from build123d import *

# Parameters (mm, degrees)
SKETCH1_R           = 2.5
BOSS_EXTRUDE1_DEPTH = 25
SKETCH2_W           = 2
SKETCH2_H           = 3
SKETCH2_W_2         = 1
SKETCH2_H_2         = 2
BOSS_EXTRUDE2_DEPTH = 4
SKETCH3_W           = 1.019035956
SKETCH3_H           = 3.229242318
CUT_EXTRUDE1_DEPTH  = 4
SKETCH4_R           = 1.3
CUT_EXTRUDE2_DEPTH  = 4
FILLET1_R           = 1
FILLET2_R           = 2
SKETCH5_R           = 0.5
BOSS_EXTRUDE3_DEPTH = 2
SKETCH6_W           = 3.503526818
SKETCH6_H           = 0.85884316
BOSS_EXTRUDE4_DEPTH = 0.5
FILLET3_R           = 0.5
SKETCH7_W           = 0.309208581
SKETCH7_H           = 0.81541506
CUT_EXTRUDE6_DEPTH  = 1
LPATTERN1_COUNT     = 2
LPATTERN1_PITCH     = 1.5
FILLET4_R           = 0.5
CUT_EXTRUDE8_DEPTH  = 1
CUT_EXTRUDE9_DEPTH  = 1
SKETCH12_R          = 0.4
BOSS_EXTRUDE5_DEPTH = 1
SKETCH13_R          = 0.4
BOSS_EXTRUDE6_DEPTH = 1


with BuildPart() as part:
    # Sketch1 → Boss-Extrude1 (new body)
    with BuildSketch(Plane(origin=(0, 0, 0), x_dir=(1, 0, 0), z_dir=(0, 1, 0))):
        with Locations(Location((0, 0, 0), (0, 0, 270))):
            Circle(SKETCH1_R)
    extrude(amount=BOSS_EXTRUDE1_DEPTH)

    # Sketch2 → Boss-Extrude2 (add)
    with BuildSketch(Plane(origin=(0, 25, 0), x_dir=(1, 0, 0), z_dir=(0, 1, 0))):
        Rectangle(SKETCH2_W, SKETCH2_H)
        Rectangle(SKETCH2_W_2, SKETCH2_H_2, mode=Mode.SUBTRACT)
    extrude(amount=BOSS_EXTRUDE2_DEPTH)

    # Sketch3 → Cut-Extrude1 (cut)
    with BuildSketch(Plane(origin=(0, 29, 0), x_dir=(1, 0, 0), z_dir=(0, 1, 0))):
        Rectangle(SKETCH3_W, SKETCH3_H)
    extrude(amount=-CUT_EXTRUDE1_DEPTH, mode=Mode.SUBTRACT)

    # Sketch4 → Cut-Extrude2 (cut)
    with BuildSketch(Plane.ZY.offset(1)):
        with Locations((0, 27)):
            Circle(SKETCH4_R)
    extrude(amount=-CUT_EXTRUDE2_DEPTH, mode=Mode.SUBTRACT)

    # Fillet1
    fillet1_edges = [part.edges().sort_by_distance(p)[0] for p in [
        (-0.754758989, 29, 1.5),
        (0.754758989, 29, -1.5),
        (-0.754758989, 29, -1.5),
        (0.754758989, 29, 1.5),
    ]]
    fillet(fillet1_edges, radius=FILLET1_R)

    # Fillet2
    # the kernel refuses this fillet: 2 mm, written as the material it takes off along each edge
    with BuildSketch(Plane(origin=(0, 0, 0), x_dir=(0, 0, 1), z_dir=(-1, 0, 0))) as fillet2_piece_1:
        with BuildLine():
            CenterArc((2.5 - FILLET2_R, FILLET2_R), FILLET2_R, 270, 90)
            Line((2.5 - FILLET2_R, 0), (2.5, 0))
            Line((2.5, 0), (2.5, FILLET2_R))
        make_face()
    revolve(axis=Axis((0, 0, 0), (0, 1, 0)), mode=Mode.SUBTRACT)
    with BuildSketch(Plane(origin=(0, 25, 0), x_dir=(0, 0, 1), z_dir=(-1, 0, 0))) as fillet2_piece_2_section:
        with BuildLine():
            CenterArc((2.5 - FILLET2_R, -FILLET2_R), FILLET2_R, 0, 90)
            Line((2.5, -FILLET2_R), (2.5, 0))
            Line((2.5, 0), (2.5 - FILLET2_R, 0))
        make_face()
    fillet2_piece_2 = revolve(axis=Axis((0, 25, 0), (0, 1, 0)), mode=Mode.PRIVATE)
    fillet2_piece_2 = split(fillet2_piece_2, bisect_by=Plane(origin=(0.509517978, 24.924108372, -1.066767337), z_dir=(-1, 0, 0)), keep=Keep.TOP, mode=Mode.PRIVATE)
    fillet2_piece_2 = split(fillet2_piece_2, bisect_by=Plane(origin=(-0.509517978, 24.924108372, -1.066767337), z_dir=(1, 0, 0)), keep=Keep.TOP, mode=Mode.PRIVATE)
    add(fillet2_piece_2, mode=Mode.SUBTRACT)
    with BuildSketch(Plane(origin=(0, 25, 0), x_dir=(0, 0, 1), z_dir=(-1, 0, 0))) as fillet2_piece_3_section:
        with BuildLine():
            CenterArc((2.5 - FILLET2_R, -FILLET2_R), FILLET2_R, 0, 90)
            Line((2.5, -FILLET2_R), (2.5, 0))
            Line((2.5, 0), (2.5 - FILLET2_R, 0))
        make_face()
    fillet2_piece_3 = revolve(axis=Axis((0, 25, 0), (0, 1, 0)), mode=Mode.PRIVATE)
    fillet2_piece_3 = split(fillet2_piece_3, bisect_by=Plane(origin=(0.753348396, 24.487146264, 1.5), z_dir=(0, 0, 1)), keep=Keep.TOP, mode=Mode.PRIVATE)
    add(fillet2_piece_3, mode=Mode.SUBTRACT)
    with BuildSketch(Plane(origin=(0, 25, 0), x_dir=(0, 0, 1), z_dir=(-1, 0, 0))) as fillet2_piece_4_section:
        with BuildLine():
            CenterArc((2.5 - FILLET2_R, -FILLET2_R), FILLET2_R, 0, 90)
            Line((2.5, -FILLET2_R), (2.5, 0))
            Line((2.5, 0), (2.5 - FILLET2_R, 0))
        make_face()
    fillet2_piece_4 = revolve(axis=Axis((0, 25, 0), (0, 1, 0)), mode=Mode.PRIVATE)
    fillet2_piece_4 = split(fillet2_piece_4, bisect_by=Plane(origin=(1, 24.532221184, 1.15e-07), z_dir=(1, 0, 0)), keep=Keep.TOP, mode=Mode.PRIVATE)
    add(fillet2_piece_4, mode=Mode.SUBTRACT)
    with BuildSketch(Plane(origin=(0, 25, 0), x_dir=(0, 0, 1), z_dir=(-1, 0, 0))) as fillet2_piece_5_section:
        with BuildLine():
            CenterArc((2.5 - FILLET2_R, -FILLET2_R), FILLET2_R, 0, 90)
            Line((2.5, -FILLET2_R), (2.5, 0))
            Line((2.5, 0), (2.5 - FILLET2_R, 0))
        make_face()
    fillet2_piece_5 = revolve(axis=Axis((0, 25, 0), (0, 1, 0)), mode=Mode.PRIVATE)
    fillet2_piece_5 = split(fillet2_piece_5, bisect_by=Plane(origin=(0.753348395, 24.487146008, -1.5), z_dir=(0, 0, -1)), keep=Keep.TOP, mode=Mode.PRIVATE)
    add(fillet2_piece_5, mode=Mode.SUBTRACT)
    with BuildSketch(Plane(origin=(0, 25, 0), x_dir=(0, 0, 1), z_dir=(-1, 0, 0))) as fillet2_piece_6_section:
        with BuildLine():
            CenterArc((2.5 - FILLET2_R, -FILLET2_R), FILLET2_R, 0, 90)
            Line((2.5, -FILLET2_R), (2.5, 0))
            Line((2.5, 0), (2.5 - FILLET2_R, 0))
        make_face()
    fillet2_piece_6 = revolve(axis=Axis((0, 25, 0), (0, 1, 0)), mode=Mode.PRIVATE)
    fillet2_piece_6 = split(fillet2_piece_6, bisect_by=Plane(origin=(-1, 24.532221184, -1.16e-07), z_dir=(-1, 0, 0)), keep=Keep.TOP, mode=Mode.PRIVATE)
    add(fillet2_piece_6, mode=Mode.SUBTRACT)

    # Sketch5 → Boss-Extrude3 (add)
    with BuildSketch(Plane(origin=(0, 0, 0), x_dir=(1, 0, 0), z_dir=(0, 1, 0))):
        with Locations(Location((0, 0, 0), (0, 0, 270))):
            Circle(SKETCH5_R)
    extrude(amount=-BOSS_EXTRUDE3_DEPTH)

    # Sketch6 → Boss-Extrude4 (add, symmetric)
    with BuildSketch(Plane.XY):
        with Locations((0, -1.427875915)):
            Rectangle(SKETCH6_W, SKETCH6_H)
    extrude(amount=BOSS_EXTRUDE4_DEPTH, both=True)

    # Fillet3
    # the kernel refuses this fillet: 0.5 mm, written as the material it takes off along each edge
    with BuildSketch(Plane(origin=(1.751763409, -0.998454335, 1.75), x_dir=(-1, 0, 0), z_dir=(0, 0, -1)), Plane(origin=(1.751763409, -1.857297495, 1.75), x_dir=(0, 1, 0), z_dir=(0, 0, -1)), Plane(origin=(-1.751763409, -0.998454335, -1.75), x_dir=(1, 0, 0), z_dir=(0, 0, 1)), Plane(origin=(-1.751763409, -1.857297495, -1.75), x_dir=(0, 1, 0), z_dir=(0, 0, 1))) as fillet3_piece_1:
        with BuildLine():
            CenterArc((FILLET3_R, -FILLET3_R), FILLET3_R, 90, 90)
            Line((0, -FILLET3_R), (0, 0))
            Line((0, 0), (FILLET3_R, 0))
        make_face()
    extrude(amount=3.5, mode=Mode.SUBTRACT)

    # Sketch7 → Cut-Extrude6 (cut)
    with BuildSketch(Plane.XZ.offset(1.857297495)):
        with Locations((-0.76394551, -0.009835432)):
            Rectangle(SKETCH7_W, SKETCH7_H)
    cut_extrude6 = extrude(amount=-CUT_EXTRUDE6_DEPTH, mode=Mode.SUBTRACT)

    # LPattern1: Cut-Extrude6 ×2
    with Locations(*[(i * LPATTERN1_PITCH, 0, 0) for i in range(1, LPATTERN1_COUNT)]):
        add(cut_extrude6, mode=Mode.SUBTRACT)

    # Fillet4
    # the kernel refuses this fillet: 0.5 mm, written as the material it adds along each edge
    # the kernel refuses this fillet: 0.5 mm, written as the material it takes off along each edge
    with BuildSketch(Plane(origin=(-0.9185498, -0.998454335, -0.417542962), x_dir=(-1, 0, 0), z_dir=(0, 0, 1)), Plane(origin=(-0.9185498, -1.857297495, -0.417542962), x_dir=(0, 1, 0), z_dir=(0, 0, 1)), Plane(origin=(0.890658781, -0.998454335, 0.397872098), x_dir=(1, 0, 0), z_dir=(0, 0, -1)), Plane(origin=(0.890658781, -1.857297495, 0.397872098), x_dir=(0, 1, 0), z_dir=(0, 0, -1))) as fillet4_2_piece_1:
        with BuildLine():
            CenterArc((FILLET4_R, FILLET4_R), FILLET4_R, 180, 90)
            Line((0, FILLET4_R), (0, 0))
            Line((0, 0), (FILLET4_R, 0))
        make_face()
    extrude(amount=0.81541506, mode=Mode.SUBTRACT)

    # Sketch10 → Cut-Extrude8 (cut)
    with BuildSketch(Plane.XZ.offset(1.857297495)):
        Polygon((-0.923556177, 0.397872098), (-1.784787166, 0.397872098), (-1.784787166, -0.417542962), (-0.876989159, -0.417542962), (-0.876989159, 0.397872098), align=None)
    extrude(amount=-CUT_EXTRUDE8_DEPTH, mode=Mode.SUBTRACT)

    # Sketch11 → Cut-Extrude9 (cut)
    with BuildSketch(Plane(origin=(0, -1.857297495, 0), x_dir=(-1, 0, 0), z_dir=(0, -1, 0))):
        Polygon((-0.741652452, -0.397872098), (-1.858092241, -0.397872098), (-1.858092241, 0.417542962), (-0.783282411, 0.417542962), align=None)
    extrude(amount=-CUT_EXTRUDE9_DEPTH, mode=Mode.SUBTRACT)

    # Sketch12 → Boss-Extrude5 (add)
    with BuildSketch(Plane.XY.offset(0.5)):
        with Locations((-1.251763409, -1.427875915)):
            Circle(SKETCH12_R)
    extrude(amount=-BOSS_EXTRUDE5_DEPTH)

    # Sketch13 → Boss-Extrude6 (add)
    with BuildSketch(Plane.XY.offset(0.5)):
        with Locations((1.251763409, -1.427875915)):
            Circle(SKETCH13_R)
    extrude(amount=-BOSS_EXTRUDE6_DEPTH)


solid = part.part
The listing builds one solid part. Answer for the finished solid, in the listing's coordinates (mm). A direction names the side the tool comes from. Round coordinates to 2 decimals unless told otherwise and drop trailing zeros. Order: outer loops, then holes, each group sorted by start corner. A loop starts at its lowest first (then second) coordinate and runs counter-clockwise, first axis right, second up. Notation, with made-up numbers: (68, 60) -> (77, 60) arc R20 cw to (77, 94) -> close; hole circle Ø5 at (-31, -5). An arc over 180 degrees is marked (long way). Put each result on its own line as item: value.
Q1. Consider line 1 along X through (y, z) = (25.5, 0.3); line 2 along X through (y, z) = (24, -1.5); line 3 along Y through (x, z) = (0.9, 0). Determine where each line is inside the solid, lowest interval first.
Results list:
line 1: -1 to -0.51, 0.51 to 1
line 2: -1.65 to 1.65
line 3: -1.62 to -1.24, 0.04 to 25.7, 28.3 to 29
Q2. Section A-A, the plane y = 27 is taken. Write down the section's boundary in (x, z), and give its area (3 significant figures).
Results list:
outline: (-1, -1.5) -> (-0.51, -1.5) -> (-0.51, -1.3) -> (-1, -1.3) -> close; (-1, 1.3) -> (-0.51, 1.3) -> (-0.51, 1.5) -> (-1, 1.5) -> close; (0.51, -1.5) -> (1, -1.5) -> (1, -1.3) -> (0.51, -1.3) -> close; (0.51, 1.3) -> (1, 1.3) -> (1, 1.5) -> (0.51, 1.5) -> close
area: 0.392 mm^2
Q3. Section B-B, the plane z = -0.95 is taken. Count the separate pieces of the cut face and the enclosed holes in it, and give its area (3 significant figures).
Results list:
separate pieces: 3
enclosed holes: 0
area: 114 mm^2
Q4. Section C-C, the plane y = 17 is taken. Write down the section's boundary in (x, z), and give its area (3 significant figures).
Results list:
outline: circle Ø5 at (0, 0)
area: 19.6 mm^2
Q5. Each of these flat-tipped pins is pushed along its axis until it touches: P1, Ø1.5, axis at y = 28, z = 0, coming from the +X side; P2, Ø1.5, axis at x = -2, z = 2, coming from the -Y side; P3, Ø0.9, axis at x = -1, y = -1.5, coming from the -Z side. Where does it stop, or does it pass through?
Results list:
P1: x = 1
P2: y = 0.77
P3: z = -0.5
Q6. Determine the mould class of faces 3 (the cylindrical face through (-0.488, -0.492, -0.108)), 4 (the cylindrical face through (0.758, 28.699, 1.215)), 5 (the flat face through (0, -1.4, 0.5)) for opening direction Y: pulls with the +Y half, pulls with the -Y half, needs draft (parallel to the pull), parting line crosses it, or undercut.
Results list:
face 3: undercut
face 4: pulls with the +Y half
face 5: needs draft
Q7. Which of the six approach directions +Z, -Z, +X, -X, +Y, -Y give full straight-line access (tool end or side, diameter ignored) to faces 1 (the flat face through (-0.609, -1.4, 0)), 2 (the cylindrical face through (-0.751, 28.699, 1.215))?
Results list:
face 1: -Y
face 2: +Z, +X, -X, +Y
